```python
from build123d import *

# Parameters (mm, degrees)
SKETCH_1_R          = 10
SKETCH_1_R_2        = 7
EXTRUDE_1_DEPTH     = 2.8
SKETCH_2_R          = 10
SKETCH_2_R_2        = 8
EXTRUDE_2_DEPTH     = 0.5
EXTRUDE_3_DEPTH     = 8.4
EXTRUDE_4_DEPTH     = 5.4
SKETCH_7_R          = 0.9
CUT_EXTRUDE_1_DEPTH = 26.870410541
CHAMFER_2_SIZE      = 2
EXTRUDE_5_REACH     = 23.757
FILLET_2_R          = 82.5
CHAMFER_4_SIZE      = 3
FILLET_3_R          = 2
CUT_EXTRUDE_START   = -7
SKETCH_9_R          = 8
CUT_EXTRUDE_2_DEPTH = 7
CHAMFER_5_SIZE      = 1


with BuildPart() as part:
    # 草图1 → 凸台-拉伸1 (new body)
    with BuildSketch(Plane(origin=(0, 0, 0), x_dir=(1, 0, 0), z_dir=(0, 1, 0))):
        with Locations(Location((0, 0, 0), (0, 0, 270))):
            Circle(SKETCH_1_R)
        with Locations(Location((0, 0, 0), (0, 0, 270))):
            Circle(SKETCH_1_R_2, mode=Mode.SUBTRACT)
    extrude(amount=EXTRUDE_1_DEPTH)

    # 草图2 → 凸台-拉伸2 (add)
    with BuildSketch(Plane(origin=(0, 2.8, 0), x_dir=(1, 0, 0), z_dir=(0, 1, 0))):
        with Locations(Location((0, 0, 0), (0, 0, 270))):
            Circle(SKETCH_2_R)
        with Locations(Location((0, 0, 0), (0, 0, 270))):
            Circle(SKETCH_2_R_2, mode=Mode.SUBTRACT)
    extrude(amount=EXTRUDE_2_DEPTH)

    # 草图3 → 凸台-拉伸3 (add)
    with BuildSketch(Plane.XZ):
        with BuildLine():
            ThreePointArc((0, 10), (-5.267826876, 8.5), (-8.95530569, 4.45))
            Line((-8.95530569, 4.45), (0, 10))
        make_face()
        with BuildLine():
            Line((8.95530569, -4.45), (0, -10))
            ThreePointArc((0, -10), (5.267826876, -8.5), (8.95530569, -4.45))
        make_face()
    extrude(amount=-EXTRUDE_3_DEPTH)

    # 草图5 → 凸台-拉伸4 (add)
    with BuildSketch(Plane(origin=(0, 8.4, 0), x_dir=(1, 0, 0), z_dir=(0, 1, 0))):
        Polygon((1.811722614, 12.923338709), (10.767028304, 7.373338709), (7.901740315, 2.75), (-1.053565375, 8.3), align=None)
        Polygon((-7.901740315, -2.75), (1.053565375, -8.3), (-1.811722614, -12.923338709), (-10.767028304, -7.373338709), align=None)
    extrude(amount=EXTRUDE_4_DEPTH)

    # 草图7 → 切除-拉伸1 (cut, through all)
    with BuildSketch(Plane(origin=(-4.477652845, 0, -2.775), x_dir=(-0.5267826876426366, 0, 0.8500000000000003), z_dir=(-0.8500000000000003, 0, -0.5267826876426366))):
        with Locations((9.219611005, 10.9)):
            Circle(SKETCH_7_R)
        with Locations((-9.219611005, 10.9)):
            Circle(SKETCH_7_R)
    extrude(amount=-CUT_EXTRUDE_1_DEPTH, mode=Mode.SUBTRACT)

    # 倒角2
    # the kernel refuses this chamfer: 2 mm, written as the material it adds along each edge
    with BuildSketch(Plane(origin=(-8.95530569, 8.4, 4.45), x_dir=(0, -1, 0), z_dir=(0.8500000000000002, 0, 0.5267826876426367))) as chamfer_2_piece_1_section:
        Polygon((CHAMFER_2_SIZE, 0), (0, CHAMFER_2_SIZE), (0, 0), align=None)
    chamfer_2_piece_1 = extrude(amount=10.535653753, mode=Mode.PRIVATE)
    chamfer_2_piece_1 = chamfer_2_piece_1 & Plane(origin=(0, 8.4, 0), x_dir=(0, 0, 1), z_dir=(0, -1, 0)) * Cylinder(10, 30, mode=Mode.PRIVATE)
    chamfer_2_piece_1 = split(chamfer_2_piece_1, bisect_by=Plane(origin=(-7.901740315, 8.4, 2.75), z_dir=(-0.5267826876426371, 0, 0.85)), keep=Keep.TOP, mode=Mode.PRIVATE)
    add(chamfer_2_piece_1)
    with BuildSketch(Plane(origin=(8.95530569, 8.4, -4.45), x_dir=(-0.5267826876426367, 0, 0.8500000000000002), z_dir=(-0.8500000000000002, 0, -0.5267826876426367))) as chamfer_2_piece_2_section:
        Polygon((CHAMFER_2_SIZE, 0), (0, -CHAMFER_2_SIZE), (0, 0), align=None)
    chamfer_2_piece_2 = extrude(amount=10.535653753, mode=Mode.PRIVATE)
    chamfer_2_piece_2 = chamfer_2_piece_2 & Plane(origin=(0, 8.4, 0), x_dir=(0, 0, -1), z_dir=(0, -1, 0)) * Cylinder(10, 30, mode=Mode.PRIVATE)
    chamfer_2_piece_2 = split(chamfer_2_piece_2, bisect_by=Plane(origin=(7.901740315, 8.4, -2.75), z_dir=(0.5267826876426374, 0, -0.8499999999999999)), keep=Keep.TOP, mode=Mode.PRIVATE)
    add(chamfer_2_piece_2)

    # 草图8 → 凸台-拉伸5 (add, up to next)
    with BuildSketch(Plane.XZ, mode=Mode.PRIVATE) as extrude_5_sk1:
        with BuildLine():
            Line((10.767028304, -7.373338709), (8.95530569, -4.45))
            ThreePointArc((8.95530569, -4.45), (5.267826876, -8.5), (0, -10))
            Line((0, -10), (1.811722614, -12.923338709))
            Line((1.811722614, -12.923338709), (10.767028304, -7.373338709))
        make_face()
    extrude_5_tool1 = extrude(extrude_5_sk1.sketch, amount=-EXTRUDE_5_REACH, mode=Mode.PRIVATE) - part.part
    # 草图8 → 凸台-拉伸5 (add, up to next)
    with BuildSketch(Plane.XZ, mode=Mode.PRIVATE) as extrude_5_sk2:
        with BuildLine():
            Line((-10.767028304, 7.373338709), (-8.95530569, 4.45))
            ThreePointArc((-8.95530569, 4.45), (-5.267826876, 8.5), (0, 10))
            Line((0, 10), (-1.811722614, 12.923338709))
            Line((-1.811722614, 12.923338709), (-10.767028304, 7.373338709))
        make_face()
    extrude_5_tool2 = extrude(extrude_5_sk2.sketch, amount=-EXTRUDE_5_REACH, mode=Mode.PRIVATE) - part.part
    add(extrude_5_tool1.solids().sort_by_distance((5.629921, 0, -9.084263))[0])
    add(extrude_5_tool2.solids().sort_by_distance((-5.629921, 0, 9.084263))[0])

    # 圆角2
    # the kernel refuses this fillet: 82.5 mm, written as the material it adds along each edge
    with BuildSketch(Plane(origin=(0, 0, -10), x_dir=(0.526782687642631, 0, -0.8500000000000036), z_dir=(0, 1, 0))) as fillet_2_piece_1:
        with BuildLine():
            CenterArc((36.184795451, 75.723030975), FILLET_2_R, 241.113318321, 5.501155307)
            ThreePointArc((-3.669211303, 3.48794154), (-1.610231073, 1.980006188), (0, 0))
            Line((0, 0), (3.43922201, 0))
        make_face()
    extrude(amount=3.3)
    with BuildSketch(Plane(origin=(8.95530569, 0, -4.45), x_dir=(0.203827060688438, 0, 0.9790069097463571), z_dir=(0, 1, 0))) as fillet_2_piece_2:
        with BuildLine():
            CenterArc((25.945282898, 79.813276697), FILLET_2_R, 249.836350841, 5.501155307)
            Line((-2.4926907, 2.369544494), (0, 0))
            ThreePointArc((0, 0), (2.531247112, 0.325663431), (5.062494224, 0))
        make_face()
    extrude(amount=3.3)
    with BuildSketch(Plane(origin=(0, 3.3, 10), x_dir=(-0.5267826876443492, 0, 0.8499999999989388), z_dir=(0, -1, 0)), Plane(origin=(-8.95530569, 0, 4.45), x_dir=(-0.5267826876426422, 0, 0.8499999999999966), z_dir=(0, 1, 0))) as fillet_2_piece_3:
        with BuildLine():
            CenterArc((36.184795451, -75.723030975), FILLET_2_R, 113.385526372, 5.501155307)
            ThreePointArc((-3.669211303, -3.48794154), (-1.610231073, -1.980006188), (0, 0))
            Line((0, 0), (3.43922201, 0))
        make_face()
    extrude(amount=3.3)

    # 倒角4
    chamfer_4_edges = [part.edges().sort_by_distance(p)[0] for p in [
        (6.289375459, 0, -10.148338709),
        (-6.289375459, 0, 10.148338709),
    ]]
    chamfer(chamfer_4_edges, length=CHAMFER_4_SIZE)

    # 圆角3
    # the kernel refuses this fillet: 2 mm, written as the material it adds along each edge
    with BuildSketch(Plane(origin=(0, 3.3, -10), x_dir=(-0.8499999999998374, 0, -0.5267826876428993), z_dir=(0.5267826876428993, 0, -0.8499999999998374))) as fillet_3_piece_1_section:
        with BuildLine():
            CenterArc((FILLET_3_R, FILLET_3_R), FILLET_3_R, 180, 90)
            Line((0, FILLET_3_R), (0, 0))
            Line((0, 0), (FILLET_3_R, 0))
        make_face()
    fillet_3_piece_1 = extrude(amount=3.43922201, mode=Mode.PRIVATE)
    fillet_3_piece_1 = fillet_3_piece_1 - Plane(origin=(-45.303052529, 3.3, -80.646657907), x_dir=(0.5267826876428993, 0, -0.8499999999998374), z_dir=(0, -1, 0)) * Cylinder(82.5, 15, mode=Mode.PRIVATE)
    add(fillet_3_piece_1)
    with BuildSketch(Plane(origin=(-8.95530569, 3.3, 4.45), x_dir=(-0.8499999999998374, 0, -0.5267826876428994), z_dir=(-0.5267826876428993, 0, 0.8499999999998374))) as fillet_3_piece_2_section:
        with BuildLine():
            CenterArc((FILLET_3_R, -FILLET_3_R), FILLET_3_R, 90, 90)
            Line((0, -FILLET_3_R), (0, 0))
            Line((0, 0), (FILLET_3_R, 0))
        make_face()
    fillet_3_piece_2 = extrude(amount=3.43922201, mode=Mode.PRIVATE)
    fillet_3_piece_2 = fillet_3_piece_2 - Plane(origin=(-92.381405818, 3.3, -4.682505639), x_dir=(-0.5267826876428993, 0, 0.8499999999998374), z_dir=(0, -1, 0)) * Cylinder(82.5, 15, mode=Mode.PRIVATE)
    add(fillet_3_piece_2)
    with BuildSketch(Plane(origin=(10.767028304, 3.3, -7.373338709), x_dir=(0.8499999999997903, 0, 0.5267826876429756), z_dir=(-0.5267826876429755, 0, 0.8499999999997901))) as fillet_3_piece_3_section:
        with BuildLine():
            CenterArc((FILLET_3_R, FILLET_3_R), FILLET_3_R, 180, 90)
            Line((0, FILLET_3_R), (0, 0))
            Line((0, 0), (FILLET_3_R, 0))
        make_face()
    fillet_3_piece_3 = extrude(amount=3.43922201, mode=Mode.PRIVATE)
    fillet_3_piece_3 = fillet_3_piece_3 - Plane(origin=(92.381405818, 3.3, 4.68250564), x_dir=(0.20382706068808945, 0, 0.9790069097464297), z_dir=(0, -1, 0)) * Cylinder(82.5, 15, mode=Mode.PRIVATE)
    add(fillet_3_piece_3)
    with BuildSketch(Plane(origin=(0, 3.3, 10), x_dir=(0.8499999999991121, 0, 0.5267826876440694), z_dir=(-0.5267826876440695, 0, 0.8499999999991122))) as fillet_3_piece_4_section:
        with BuildLine():
            CenterArc((FILLET_3_R, FILLET_3_R), FILLET_3_R, 180, 90)
            Line((0, FILLET_3_R), (0, 0))
            Line((0, 0), (FILLET_3_R, 0))
        make_face()
    fillet_3_piece_4 = extrude(amount=3.43922201, mode=Mode.PRIVATE)
    fillet_3_piece_4 = fillet_3_piece_4 - Plane(origin=(45.303052529, 3.3, 80.646657907), x_dir=(-0.5267826876440695, 0, 0.8499999999991122), z_dir=(0, 1, 0)) * Cylinder(82.5, 15, mode=Mode.PRIVATE)
    add(fillet_3_piece_4)

    # 草图9 → 切除-拉伸2 (cut)
    with BuildSketch(Plane(origin=(0, 13.8, 0), x_dir=(1, 0, 0), z_dir=(0, 1, 0)).offset(CUT_EXTRUDE_START)):
        with Locations(Location((0, 0, 0), (0, 0, 270))):
            Circle(SKETCH_9_R)
    extrude(amount=CUT_EXTRUDE_2_DEPTH, mode=Mode.SUBTRACT)

    # 倒角5
    chamfer_5_edges = [part.edges().sort_by_distance(p)[0] for p in [
        (-8.5, 3.3, -5.267826876),
        (8.5, 3.3, 5.267826876),
        (-10.117707279, 3.3, 1.557198087),
        (10.117707279, 3.3, -1.557198087),
        (3.10786125, 3.3, 9.753669305),
        (-3.10786125, 3.3, -9.753669305),
    ]]
    chamfer(chamfer_5_edges, length=CHAMFER_5_SIZE)


solid = part.part
```
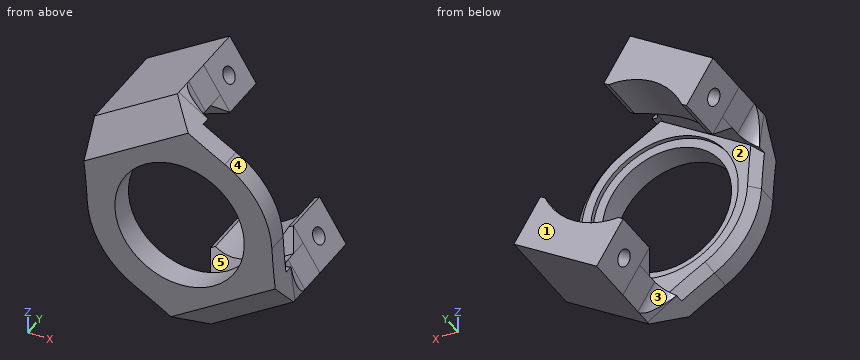
Input: part model. Units: mm. Frame: model coordinates. Face numbers are marked on the shaded views. A direction names the side the tool comes from. Give positions to 0.01 mm unless a question says otherwise; leave off trailing zeros. Put each result on its own line as item: value.
Item 1: Section query A-A, the plane x = -2.25. Count the separate pieces of the cut face and the enclosed holes in it, then the cut area to 3 significant figures.
Found:
separate pieces: 2
enclosed holes: 1
area: 71.0 mm^2
Item 2: Access query for the marked faces 4 and 5. Directions: +Z, -Z, +X, -X, +Y, -Y. A direction counts if a zero-diameter tool reaches every point of the face in a straight line with its end or side. Return the directions, or none.
Found:
face 4: +Z, +X, +Y, -Y
face 5: -X
Item 3: Draft query along Z for the marked faces 1, 2 and 3. Return one class per face: +Z half, -Z half, draft (parallel to the pull), parting line (faces both ways), or undercut.
Found:
face 1: draft
face 2: undercut
face 3: -Z half
Item 4: Contact query for flat-ended pins moving along their axis: pin 1 (2 mm diameter, centred on x = -6.5, y = 7, fed in from +Z); pin 2 (3 mm diameter, centred on x = 8, y = 10.5, fed in from +Z); pin 3 (6 mm diameter, centred on y = 7.5, z = 8, fed in from +X); pin 4 (2 mm diameter, centred on x = 3.5, z = 2, fed in from +Y). Output: stop coordinate, or through.
Found:
pin 1: stops at z = 10.64
pin 2: stops at z = -2.75
pin 3: stops at x = 1.05
pin 4: passes through
Item 5: Ray query, L1, parallel to Y at x = 4.5, z = 6.5; L2, parallel to X at y = 1.5, z = -2.5; L3, parallel to X at y = 3.2, z = 0. Return the intervals inside material, ascending. Write a range as from..to.
Found:
L1: y = 0..2.8
L2: x = -9.68..-6.54, 6.54..10.19
L3: x = -9.11..-8, 8..9.11
